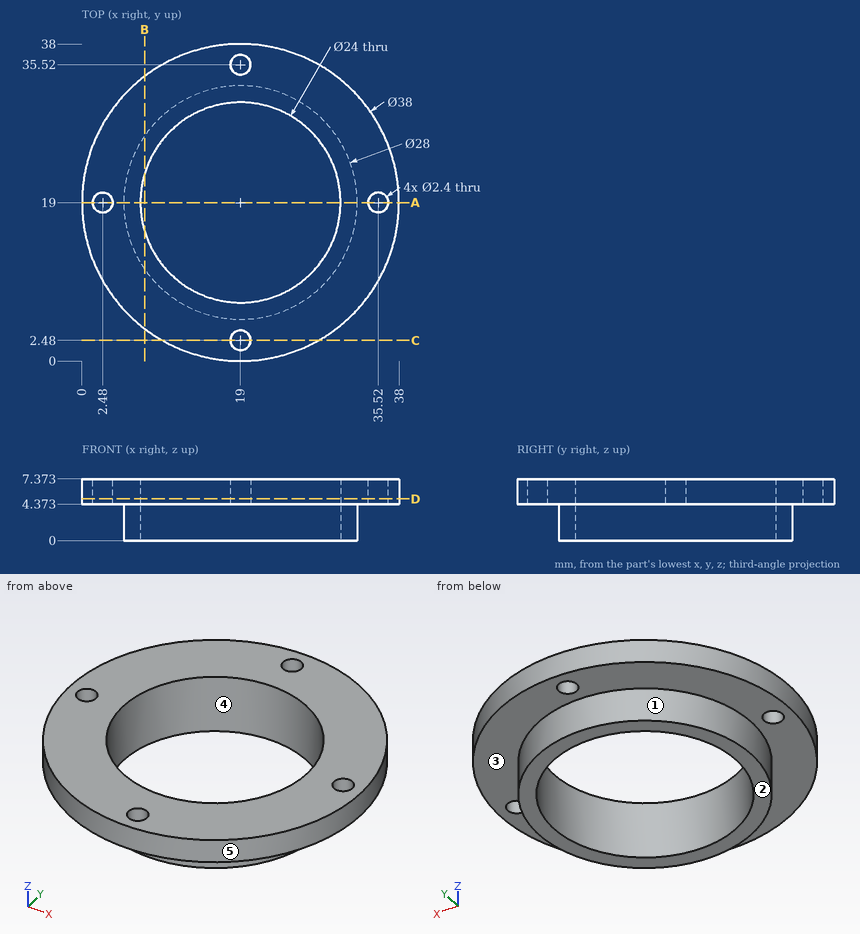
Check sheet for the drawn part. Datum: minimum x, y, z corner. Units: mm. A direction names the side the tool comes from. Coordinates: 2 decimals unless noted, no trailing zeros. Loops run counter-clockwise (first coordinate to the right, second up) from the corner with the lowest first, then second, coordinate; pieces in that order, holes last. Notation, with made-up numbers: M 17,49 L 29,49 A19 ccw 29,67 Z; hole C 58,64 d4. An arc over 180 degrees is marked long. Answer as a JSON object with one key per item and string values.
1. Access from +Z, -Z, +X, -X, +Y, -Y to the whole of each face (thin tool, end or side, straight path). Record for the marked faces 1 and 2.
Outcome:
{"face 1": "-Z", "face 2": "-Z, +X, -X, +Y, -Y"}
2. Scan lines: L1, parallel to Y at x = 19, z = 5.8; L2, parallel to Y at x = 19, z = 2; L3, parallel to X at y = 35.5, z = 5.5 (1 decimal). Record each from-to range of solid material in increasing order. Write a range as from..to.
Outcome:
{"L1": "0..1.28, 3.68..7, 31..34.32, 36.72..38", "L2": "5..7, 31..33", "L3": "9.6..17.8, 20.2..28.4"}
3. Depth check by flat-ended pin: P1, Ø4, axis at x = 16.5, z = 5, coming from the +Y side; P2, Ø3, axis at x = 19, y = 35.52, coming from the -Z side; P3, Ø2, axis at y = 12.5, z = 6, coming from the +X side. Enter the tip coordinate at first touch or a pass-through.
Outcome:
{"P1": "y = 37.99", "P2": "z = 4.37", "P3": "x = 37.19"}
4. Release check for a two-part mould opening along X. For the marked faces 3, 4 and 5 record: pulls with the +X half, pulls with the -X half, needs draft (parallel to the pull), parting line crosses it, or undercut.
Outcome:
{"face 3": "needs draft", "face 4": "undercut", "face 5": "parting line crosses it"}
5. Sectioned sample at B-B on x = 7.5. Record the cut outline in (y, z) (1 decimal).
Outcome:
{"outline": "M 3.9,4.4 L 11,4.4 L 11,0 L 15.6,0 L 15.6,7.4 L 3.9,7.4 Z; M 22.4,0 L 27,0 L 27,4.4 L 34.1,4.4 L 34.1,7.4 L 22.4,7.4 Z"}
6. Sectioned sample at D-D on z = 5. Record the cut outline in (x, y).
Outcome:
{"outline": "C 19,19 d38; hole C 2.48,19 d2.4; hole C 19,19 d24; hole C 19,2.48 d2.4; hole C 19,35.52 d2.4; hole C 35.52,19 d2.4"}
7. Sectioned sample at C-C on y = 2.48. Record the cut outline in (x, z) (1 decimal).
Outcome:
{"outline": "M 9.6,4.4 L 17.8,4.4 L 17.8,7.4 L 9.6,7.4 Z; M 20.2,4.4 L 28.4,4.4 L 28.4,7.4 L 20.2,7.4 Z"}
8. Sectioned sample at A-A on y = 19. Record the cut outline in (x, z).
Outcome:
{"outline": "M 0,4.37 L 1.28,4.37 L 1.28,7.37 L 0,7.37 Z; M 3.68,4.37 L 5,4.37 L 5,0 L 7,0 L 7,7.37 L 3.68,7.37 Z; M 31,0 L 33,0 L 33,4.37 L 34.32,4.37 L 34.32,7.37 L 31,7.37 Z; M 36.72,4.37 L 38,4.37 L 38,7.37 L 36.72,7.37 Z"}
